Geometry check sheet. Reference: the model listing, model coordinates, mm. Give positions to 0.01 mm unless a question says otherwise; leave off trailing zeros. Write each loop counter-clockwise with the first axis right and the second up, starting at its lowest first coordinate (ties: lowest second). Pieces come first, ordered by that corner, then holes. Notation, with made-up numbers: (36.5, 81) -> (94.5, 81) arc R34 ccw to (94.5, 114) -> close; hole circle Ø3 at (58, 38). An arc over 180 degrees is marked (long way). One line per item, written item: value.
from build123d import *

# Parameters (mm, degrees)
F1_DEPTH = 3.175
F2_R     = 25.617872
F3_DEPTH = 0.0254


with BuildPart() as f1:
    # F0 (on Top) → F1 (new body)
    with BuildSketch(Plane.XY):
        Polygon((63.379409, 66.106962), (50.639269, 88.080784), (25.239311, 88.034409), (-0.160646, 87.988034), (-25.560604, 87.94166), (-50.960562, 87.895285), (-63.620379, 65.875089), (-76.280196, 43.854893), (-88.940013, 21.834698), (-101.599831, -0.185498), (-88.85969, -22.15932), (-76.11955, -44.133141), (-63.379409, -66.106962), (-50.639269, -88.080784), (-25.239311, -88.034409), (0.160646, -87.988034), (25.560604, -87.94166), (50.960562, -87.895285), (63.620379, -65.875089), (76.280196, -43.854893), (88.940013, -21.834698), (101.599831, 0.185498), (88.85969, 22.15932), (76.11955, 44.133141), align=None)
        Polygon((-76.280196, 43.854893), (-63.620379, 65.875089), (-66.372903, 67.457566), (-79.032721, 45.437371), align=None)
        Polygon((-101.599831, -0.185498), (-88.940013, 21.834698), (-91.692538, 23.417175), (-103.438712, 2.98615), align=None)
        Polygon((-50.960562, 87.895285), (-25.560604, 87.94166), (-25.566401, 91.116654), (-49.133274, 91.073627), align=None)
        Polygon((-0.160646, 87.988034), (25.239311, 88.034409), (25.233515, 91.209404), (-0.166443, 91.163029), align=None)
        Polygon((54.305437, 88.087477), (50.639269, 88.080784), (63.379409, 66.106962), (66.126137, 67.69948), align=None)
        Polygon((78.866278, 45.725658), (76.11955, 44.133141), (88.85969, 22.15932), (91.606418, 23.751837), align=None)
        Polygon((103.438712, -2.98615), (101.599831, 0.185498), (88.940013, -21.834698), (91.692538, -23.417175), align=None)
        Polygon((79.032721, -45.437371), (76.280196, -43.854893), (63.620379, -65.875089), (66.372903, -67.457566), align=None)
        Polygon((49.133274, -91.073627), (50.960562, -87.895285), (25.560604, -87.94166), (25.566401, -91.116654), align=None)
        Polygon((0.166443, -91.163029), (0.160646, -87.988034), (-25.239311, -88.034409), (-25.233515, -91.209404), align=None)
        Polygon((-50.639269, -88.080784), (-63.379409, -66.106962), (-66.126137, -67.69948), (-54.305437, -88.087477), align=None)
        Polygon((-76.11955, -44.133141), (-88.85969, -22.15932), (-91.606418, -23.751837), (-78.866278, -45.725658), align=None)
    extrude(amount=F1_DEPTH)

    # F2 (on face) → F3 (join)
    with BuildSketch(Plane.XY.offset(3.175)):
        Circle(F2_R)
    extrude(amount=F3_DEPTH)


solid = f1.part
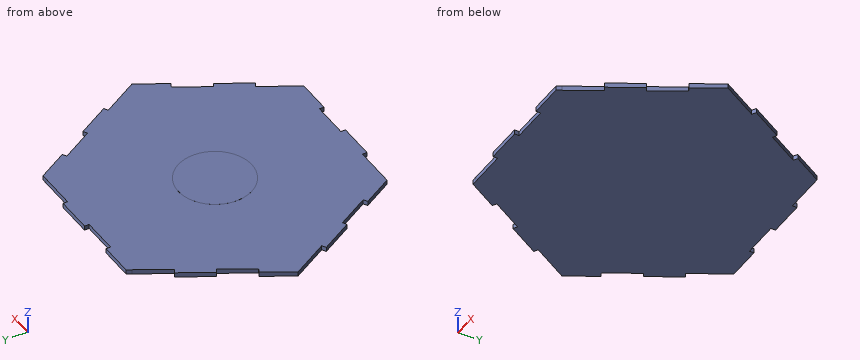
1) Sectioned sample at B-B on x = 83. Record the cut outline in (y, z) (3 decimals), plus the area to 3 significant figures.
Verdict:
outline: (-32.167, 0) -> (38.596, 0) -> (38.596, 3.175) -> (-32.167, 3.175) -> close
area: 225 mm^2
2) Sectioned sample at A-A on y = -62.5. Record the cut outline in (x, z) (3 decimals).
Verdict:
outline: (-65.471, 0) -> (69.223, 0) -> (69.223, 3.175) -> (-65.471, 3.175) -> close
3) Scan lines: probe 1 along Z at (x, y) = (-53, -57) (3 decimals); probe 2 along Y at (x, z) = (9.5, 1.95); probe 3 along Y at (x, z) = (91, 1.3). Record each from-to range of solid material in increasing order.
Verdict:
probe 1: 0 to 3.175
probe 2: -87.97 to 91.18
probe 3: -23.02 to 18.47, 23.4 to 24.8
